Input: dimensioned drawing with shaded views. Units: mm. Origin: part minimum x, y, z. A direction names the side the tool comes from. Coordinates: 2 decimals unless noted, no trailing zeros. Write each loop counter-clockwise with the first axis right and the second up, starting at its lowest first coordinate (ties: lowest second). Pieces come first, ordered by that corner, then holes. Notation, with made-up numbers: M 47.25,49.5 L 94.25,49.5 A20 cw 94.25,55.5 Z; hole C 89.25,-39.75 d10. An arc over 180 degrees is marked long. Use one line per item in the form item = value.
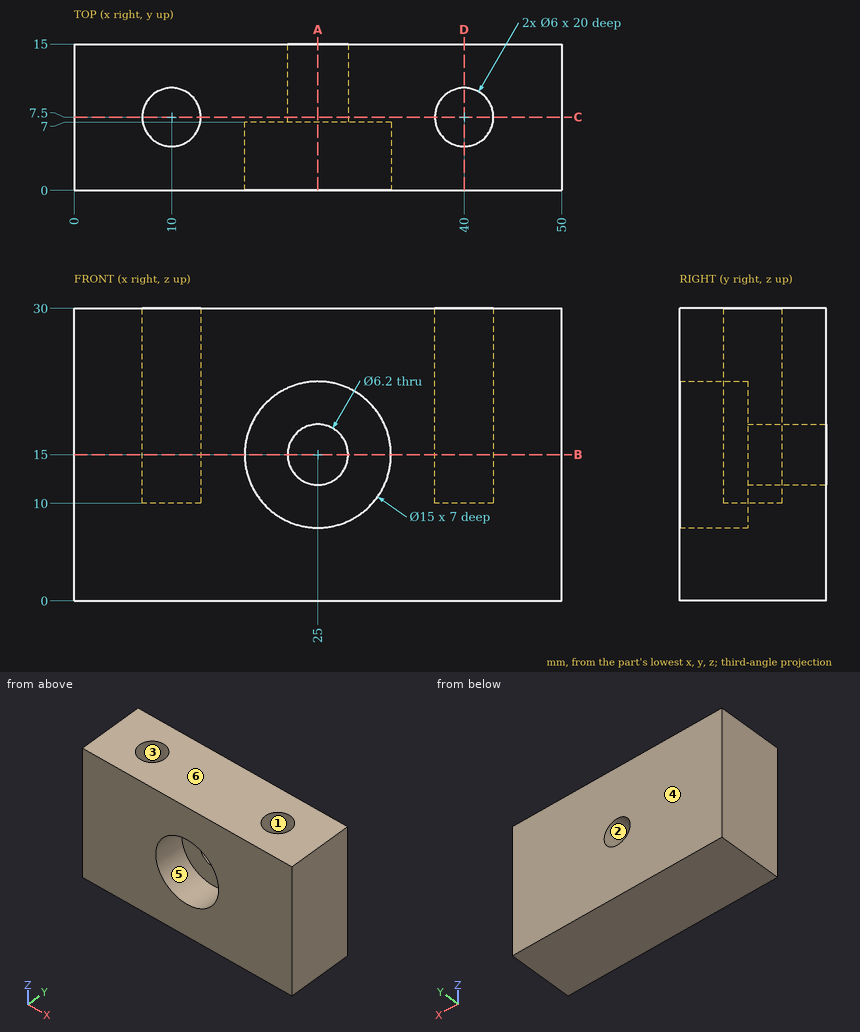
(1) Section query C-C on y = 7.5. Return the cut outline in (x, z).
Computed:
outline = M 0,0 L 50,0 L 50,30 L 43,30 L 43,10 L 37,10 L 37,30 L 13,30 L 13,10 L 7,10 L 7,30 L 0,30 Z; hole C 25,15 d6.2
(2) Set-up query: the marked faces 5 and 6. Return all of +Z, -Z, +X, -X, +Y, -Y with unobstructed straight access to the full face (end or side cutting, diameter ignored); none if empty.
Computed:
face_5 = -Y
face_6 = +Z, +X, -X, +Y, -Y
(3) Section query D-D on x = 40. Return the cut outline in (y, z).
Computed:
outline = M 0,0 L 15,0 L 15,30 L 10.5,30 L 10.5,10 L 4.5,10 L 4.5,30 L 0,30 Z
(4) Section query A-A on x = 25. Return the cut outline in (y, z), plus the area to 3 significant figures.
Computed:
outline = M 0,0 L 15,0 L 15,11.9 L 7,11.9 L 7,7.5 L 0,7.5 Z; M 0,22.5 L 7,22.5 L 7,18.1 L 15,18.1 L 15,30 L 0,30 Z
area = 295 mm^2
(5) Pull-direction query (Y, two-part tool) for the marked faces 1, 2, 3 and 4; classes: pulls with the +Y half, pulls with the -Y half, needs draft (parallel to the pull), parting line crosses it, or undercut.
Computed:
face_1 = undercut
face_2 = needs draft
face_3 = undercut
face_4 = pulls with the +Y half
(6) First-contact query: pin 1 Ø1 at (x, z) = (22, 12.5) entering from -Y; pin 2 Ø3.5 at (x, y) = (40, 7.5) entering from +Z. Flat tips, straight axial feed; report the tip coordinate or a pass-through.
Computed:
pin_1 = 7
pin_2 = 10
(7) Line query: probe 1 along Z at (x, y) = (25, 3); probe 2 along X at (y, z) = (9.5, 29); probe 3 along Y at (x, z) = (10, 15.5). Output: solid intervals per line, ascending.
Computed:
probe_1 = 0 to 7.5, 22.5 to 30
probe_2 = 0 to 7.76, 12.24 to 37.76, 42.24 to 50
probe_3 = 0 to 4.5, 10.5 to 15
(8) Section query B-B on z = 15. Return the cut outline in (x, y).
Computed:
outline = M 0,0 L 17.5,0 L 17.5,7 L 21.9,7 L 21.9,15 L 0,15 Z; M 28.1,7 L 32.5,7 L 32.5,0 L 50,0 L 50,15 L 28.1,15 Z; hole C 10,7.5 d6; hole C 40,7.5 d6
